```python
from build123d import *

# Parameters (mm, degrees)
SKETCH_1_R          = 2
SKETCH_1_R_2        = 1.5
SKETCH_1_R_3        = 1.4
SKETCH_1_W          = 42
SKETCH_1_H          = 42
SKETCH_1_W_2        = 17
SKETCH_1_H_2        = 19
EXTRUDE_1_DEPTH     = 1.2
SKETCH_2_R          = 2.5
SKETCH_2_R_2        = 1.5
SKETCH_2_W          = 31
SKETCH_2_H          = 66
SKETCH_2_W_2        = 29
SKETCH_2_H_2        = 64
EXTRUDE_2_DEPTH     = 5
SKETCH_3_W          = 15
SKETCH_3_H          = 3
CUT_EXTRUDE_1_DEPTH = 5


with BuildPart() as part:
    # 草图1 → 凸台-拉伸1 (new body)
    with BuildSketch(Plane(origin=(0, 0, 0), x_dir=(1, 0, 0), z_dir=(0, 1, 0))):
        Polygon((104.4, 68), (125.6, 68), (125.6, 100), (0, 100), (0, 0), (104.4, 0), align=None)
        with Locations(Location((5, 5, 0), (0, 0, 270))):
            Circle(SKETCH_1_R, mode=Mode.SUBTRACT)
        with Locations(Location((5, 95, 0), (0, 0, 90))):
            Circle(SKETCH_1_R, mode=Mode.SUBTRACT)
        with Locations(Location((120.6, 95, 0), (0, 0, 270))):
            Circle(SKETCH_1_R, mode=Mode.SUBTRACT)
        with Locations(Location((99.4, 5, 0), (0, 0, 90))):
            Circle(SKETCH_1_R, mode=Mode.SUBTRACT)
        with Locations(Location((101.4, 12.5, 0), (0, 0, 270))):
            Circle(SKETCH_1_R_2, mode=Mode.SUBTRACT)
        with Locations(Location((77.4, 12.5, 0), (0, 0, 90))):
            Circle(SKETCH_1_R_2, mode=Mode.SUBTRACT)
        with Locations(Location((101.4, 59.5, 0), (0, 0, 270))):
            Circle(SKETCH_1_R_2, mode=Mode.SUBTRACT)
        with Locations(Location((77.4, 59.5, 0), (0, 0, 90))):
            Circle(SKETCH_1_R_2, mode=Mode.SUBTRACT)
        with Locations(Location((60.2, 8, 0), (0, 0, 270))):
            Circle(SKETCH_1_R_3, mode=Mode.SUBTRACT)
        with Locations(Location((44.2, 8, 0), (0, 0, 90))):
            Circle(SKETCH_1_R_3, mode=Mode.SUBTRACT)
        with Locations((52.2, 67)):
            Rectangle(SKETCH_1_W, SKETCH_1_H, mode=Mode.SUBTRACT)
        with Locations((89.4, 25.5)):
            Rectangle(SKETCH_1_W_2, SKETCH_1_H_2, mode=Mode.SUBTRACT)
    extrude(amount=EXTRUDE_1_DEPTH)

    # 草图2 → 凸台-拉伸2 (add)
    # profile 1 of 3: a face of its own
    with BuildSketch(Plane(origin=(0, 1.2, 0), x_dir=(1, 0, 0), z_dir=(0, 1, 0))):
        with Locations(Location((12.5, 11.5, 0), (0, 0, 90))):
            Circle(SKETCH_2_R)
        with Locations(Location((12.5, 11.5, 0), (0, 0, 270))):
            Circle(SKETCH_2_R_2, mode=Mode.SUBTRACT)
    # profile 2 of 3: a face of its own
    with BuildSketch(Plane(origin=(0, 1.2, 0), x_dir=(1, 0, 0), z_dir=(0, 1, 0))):
        with Locations(Location((5.7, 11.5, 0), (0, 0, 90))):
            Circle(SKETCH_2_R)
        with Locations(Location((5.7, 11.5, 0), (0, 0, 270))):
            Circle(SKETCH_2_R_2, mode=Mode.SUBTRACT)
    # profile 3 of 3: a face of its own
    with BuildSketch(Plane(origin=(0, 1.2, 0), x_dir=(1, 0, 0), z_dir=(0, 1, 0))):
        with Locations((15.7, 57)):
            Rectangle(SKETCH_2_W, SKETCH_2_H)
        with Locations((15.7, 57)):
            Rectangle(SKETCH_2_W_2, SKETCH_2_H_2, mode=Mode.SUBTRACT)
    extrude(amount=EXTRUDE_2_DEPTH)

    # 草图3 → 切除-拉伸1 (cut)
    with BuildSketch(Plane(origin=(0, 6.2, 0), x_dir=(1, 0, 0), z_dir=(0, 1, 0))):
        with Locations((9.7, 25.5)):
            Rectangle(SKETCH_3_W, SKETCH_3_H)
    extrude(amount=-CUT_EXTRUDE_1_DEPTH, mode=Mode.SUBTRACT)


solid = part.part
```
Model file for the job. Use its own axes, mm. A direction names the side the tool comes from. Give positions to 0.01 mm unless a question says otherwise; leave off trailing zeros. Write each loop counter-clockwise with the first axis right and the second up, starting at its lowest first coordinate (ties: lowest second). Pieces come first, ordered by that corner, then holes. Notation, with made-up numbers: M 36.5,-21 L 56.5,-21 A11 cw 56.5,0 Z; hole C 43.25,65.5 d11. An arc over 180 degrees is marked long. Use a Markdown table: item, result.
1) Pin check, flat tips, straight feed: pin 1 (2.5 mm diameter, centred on x = 24.5, y = 3.5, fed in from +Z); pin 2 (1 mm diameter, centred on x = 40.5, z = -36, fed in from +Y); pin 3 (3 mm diameter, centred on x = 19, y = 3.5, fed in from -Z). Stop position of each tip, or through.
Responses:
| item | result |
|---|---|
| pin 1 | stops at z = -24 |
| pin 2 | stops at y = 1.2 |
| pin 3 | stops at z = -90 |
2) Drill centre lines: line 1 (X direction, y = 0.9, z = -12.5); line 2 (Z direction, x = 77.4, y = 0.95); line 3 (X direction, y = 3.5, z = -11.5). Where is each one in solid material? Low to high. Write a range as from..to.
Responses:
| item | result |
|---|---|
| line 1 | x = 0..75.9, 78.9..99.9, 102.9..104.4 |
| line 2 | z = -100..-61, -58..-14, -11..0 |
| line 3 | x = 3.2..4.2, 7.2..8.2, 10..11, 14..15 |
3) Pull direction Z, two halves, no side cores. Call faces 4 (the cylindrical face through (5.6, 3.7, -9)), 5 (the flat face through (31, 6.2, -57)), 6 (the flat face through (15, 4, -90)): +Z half, -Z half, draft (parallel to the pull), parting line (faces both ways), or undercut.
Responses:
| item | result |
|---|---|
| face 4 | undercut |
| face 5 | draft |
| face 6 | -Z half |
4) Cut at C-C (x = 35.5). List the corners of the cut face in (y, z), and give its area (3 significant figures).
Responses:
| item | result |
|---|---|
| outline | M 0,-100 L 1.2,-100 L 1.2,-88 L 0,-88 Z; M 0,-46 L 1.2,-46 L 1.2,0 L 0,0 Z |
| area | 69.6 mm2 |
5) Cut at D-D (z = -95). List the corners of the cut face in (x, y).
Responses:
| item | result |
|---|---|
| outline | M 0,0 L 3,0 L 3,1.2 L 0,1.2 Z; M 7,0 L 118.6,0 L 118.6,1.2 L 7,1.2 Z; M 122.6,0 L 125.6,0 L 125.6,1.2 L 122.6,1.2 Z |
6) Cut at B-B (y = 2.5). List the corners of the cut face in (x, z).
Responses:
| item | result |
|---|---|
| outline | M 0.2,-90 L 31.2,-90 L 31.2,-24 L 17.2,-24 L 17.2,-25 L 30.2,-25 L 30.2,-89 L 1.2,-89 L 1.2,-25 L 2.2,-25 L 2.2,-24 L 0.2,-24 Z; C 5.7,-11.5 d5; C 12.5,-11.5 d5; hole C 5.7,-11.5 d3; hole C 12.5,-11.5 d3 |
7) Tool access for faces 1 (the cylindrical face through (12.57, 3.66, -13)), 2 (the flat face through (0.2, 4, -57)), 3 (the cylindrical face through (100.07, 0.59, -58.81)): list every direction of +Z, -Z, +X, -X, +Y, -Y with a clear straight run to the whole face (end or side of a thin tool).
Responses:
| item | result |
|---|---|
| face 1 | +Y |
| face 2 | +Z, -Z, -X, +Y |
| face 3 | +Y, -Y |
8) Cut at A-A (z = -59.5). List the corners of the cut face in (x, y).
Responses:
| item | result |
|---|---|
| outline | M 0,0 L 31.2,0 L 31.2,6.2 L 30.2,6.2 L 30.2,1.2 L 1.2,1.2 L 1.2,6.2 L 0.2,6.2 L 0.2,1.2 L 0,1.2 Z; M 73.2,0 L 75.9,0 L 75.9,1.2 L 73.2,1.2 Z; M 78.9,0 L 99.9,0 L 99.9,1.2 L 78.9,1.2 Z; M 102.9,0 L 104.4,0 L 104.4,1.2 L 102.9,1.2 Z |
